For this review, take the finished solid that the model builds, in its own axes (mm). A direction names the side the tool comes from. Coordinates: 2 decimals unless noted, no trailing zeros. Loops run counter-clockwise (first coordinate to the right, second up) from the corner with the lowest first, then second, coordinate; pieces in that order, holes last. Notation, with made-up numbers: M -2.75,58.5 L 35.25,58.5 A20 cw 35.25,66.5 Z; hole C 10.25,15.5 d11. An arc over 180 degrees is marked long. Use one line per item in the form item = value.
```python
from build123d import *

# Parameters (mm, degrees)
ESBO_O1_W                       = 44
ESBO_O1_H                       = 38
RESSALTO_EXTRUS_O1_DEPTH        = 72
ESBO_O2_R                       = 15.5
CORTE_EXTRUS_O1_DEPTH           = 66
ESBO_O4_R                       = 9
CORTE_EXTRUS_O2_DEPTH           = 88.954533709
FURO_ROSCADO_DE_M51_D           = 4.2
FURO_ROSCADO_DE_M51_DEPTH       = 16.7381927
FURO_ROSCADO_DE_M51_CSINK_D     = 5.05
FURO_ROSCADO_DE_M51_CSINK_ANGLE = 90
FURO_ROSCADO_DE_M51_TIP         = 1.2618073
CHANFRO1_SIZE                   = 3
ESBO_O7_W                       = 15
ESBO_O7_H                       = 1
CORTE_EXTRUS_O3_DEPTH           = 93.54188241


with BuildPart() as part:
    # Esboço1 → Ressalto-extrusão1 (new body)
    with BuildSketch(Plane(origin=(0, 0, 0), x_dir=(0, 0, -1), z_dir=(1, 0, 0))):
        with Locations((22, 19)):
            Rectangle(ESBO_O1_W, ESBO_O1_H)
    extrude(amount=-RESSALTO_EXTRUS_O1_DEPTH)

    # Esboço2 → Corte-extrusão1 (cut)
    with BuildSketch(Plane(origin=(0, 0, 0), x_dir=(0, 0, -1), z_dir=(1, 0, 0))):
        with Locations((22, 17)):
            Circle(ESBO_O2_R)
    extrude(amount=-CORTE_EXTRUS_O1_DEPTH, mode=Mode.SUBTRACT)

    # Esboço4 → Corte-extrusão2 (cut, through all)
    with BuildSketch(Plane(origin=(-66, 0, 0), x_dir=(0, 0, -1), z_dir=(1, 0, 0))):
        with Locations((22, 17)):
            Circle(ESBO_O4_R)
    extrude(amount=-CORTE_EXTRUS_O2_DEPTH, mode=Mode.SUBTRACT)

    # Furo roscado de M51
    with Locations(Plane(origin=(0, 0, 0), x_dir=(0, 0, -1), z_dir=(1, 0, 0))):
        with Locations((8.5, 31), (35.5, 31), (38, 7), (6, 7)):
            CounterSinkHole(FURO_ROSCADO_DE_M51_D / 2, FURO_ROSCADO_DE_M51_CSINK_D / 2, depth=FURO_ROSCADO_DE_M51_DEPTH, counter_sink_angle=FURO_ROSCADO_DE_M51_CSINK_ANGLE)
            with Locations((0, 0, -(FURO_ROSCADO_DE_M51_DEPTH + FURO_ROSCADO_DE_M51_TIP / 2))):  # 118° drill point
                Cone(0, FURO_ROSCADO_DE_M51_D / 2, FURO_ROSCADO_DE_M51_TIP, mode=Mode.SUBTRACT)

    # Chanfro1
    chanfro1_edges = [part.edges().sort_by_distance(p)[0] for p in [
        (-36, 0, -44),
        (-36, 0, 0),
    ]]
    chamfer(chanfro1_edges, length=CHANFRO1_SIZE)

    # Esboço7 → Corte-extrusão3 (cut, through all)
    with BuildSketch(Plane(origin=(0, 0, 0), x_dir=(0, 0, -1), z_dir=(1, 0, 0))):
        with Locations((22, 37.5)):
            Rectangle(ESBO_O7_W, ESBO_O7_H)
    extrude(amount=-CORTE_EXTRUS_O3_DEPTH, mode=Mode.SUBTRACT)


solid = part.part
```
1. Consider section D-D on x = -38.5. Write out the cut boundary in (y, z).
Computed values:
outline = M 0,-41 L 3,-44 L 38,-44 L 38,-29.5 L 37,-29.5 L 37,-14.5 L 38,-14.5 L 38,0 L 3,0 L 0,-3 Z; hole C 17,-22 d31
2. Consider section A-A on z = -22. Write out the cut boundary in (x, y), plus the area to 3 significant figures.
Computed values:
outline = M -72,0 L 0,0 L 0,1.5 L -66,1.5 L -66,8 L -72,8 Z; M -72,26 L -66,26 L -66,32.5 L 0,32.5 L 0,37 L -72,37 Z
area = 510 mm2
3. Draft analysis for pull direction Y (two halves, no side actions). For faces 4 (the face through (-35, 38, -7)), 5 (the face through (-35, 0, -22)), 6 (the face through (-18, 7, -38)), 7 (the face through (-72, 28, -22)), state which applies: +Y half, -Y half, draft (parallel to the pull), parting line (faces both ways), or undercut.
Computed values:
face_4 = +Y half
face_5 = -Y half
face_6 = undercut
face_7 = draft
4. Wall thickness on line 1 along Z through (x, y) = (-5, 31); line 2 along Y through (x, z) = (-12.25, -38); line 3 along X through (y, z) = (3.5, -21): over which ranges is each line inside the solid? List them lowest first. Write a range as from..to.
Computed values:
line_1 = -44..-37.6, -33.4..-28.65, -15.35..-10.6, -6.4..0
line_2 = 0..4.9, 9.1..38
line_3 = -72..-66
5. Tool access review of faces 1 (the face through (0, 32, -17)), 2 (the face through (-8.696, 29.722, -37.166)), 3 (the face through (-35, 37, -22)): name each direction out of +Z, -Z, +X, -X, +Y, -Y from which nothing blocks a thin tool from reaching the whole face with its end or side.
Computed values:
face_1 = +Z, -Z, +X, +Y, -Y
face_2 = +X
face_3 = +X, -X, +Y
6. Consider section C-C on x = -6.5. Write out the cut boundary in (y, z), plus the area to 3 significant figures.
Computed values:
outline = M 0,-41 L 3,-44 L 38,-44 L 38,-29.5 L 37,-29.5 L 37,-14.5 L 38,-14.5 L 38,0 L 3,0 L 0,-3 Z; hole C 17,-22 d31; hole C 7,-38 d4.2; hole C 7,-6 d4.2; hole C 31,-35.5 d4.2; hole C 31,-8.5 d4.2
area = 838 mm2
7. Consider section B-B on y = 17. Write out the cut boundary in (x, z).
Computed values:
outline = M -72,-44 L 0,-44 L 0,-37.5 L -66,-37.5 L -66,-31 L -72,-31 Z; M -72,-13 L -66,-13 L -66,-6.5 L 0,-6.5 L 0,0 L -72,0 Z
8. For pin 1 Ø5 at (y, z) = (31, -8.5) entering from +X (3 decimals); pin 2 Ø2.5 at (y, z) = (31, -35.5) entering from +X; pin 3 Ø7.5 at (x, z) = (-31.5, -20) entering from +Y, all flat-tipped, find the tip position at first contact; note any pin that passes through.
Computed values:
pin_1 = -0.025
pin_2 = -17.25
pin_3 = 37
